Can you work these out from the model? Positions are in its coordinate system, mm. A direction names the side the tool comes from. Give positions to 0.01 mm unless a question says otherwise; leave off trailing zeros. Order: outer loops, then holes, each group sorted by start corner. A loop starts at its lowest first (then second) coordinate and runs counter-clockwise, first axis right, second up. Notation, with made-up numbers: M -6.5,13.5 L 50.5,13.5 A30 cw 50.5,35.5 Z; hole C 0,-32.75 d5. An arc over 180 degrees is marked long. Answer as a JSON object with one key per item and string values.
Autodesk Inventor part; units mm, degrees
ref_plane "Work Plane1" through (-19.6075, -25, -15) normal (0, 0, 1) x (1, 0, 0)
ref_plane "Work Plane2" through (-137.3725, -100, -40) normal (0, 0, -1) x (0, 1, 0)
ref_plane "Work Plane3" through (-19.6075, -25, -15) normal (0, 0, 1) x (1, 0, 0)
sketch "Sketch1" plane through (0, 0, 0) normal (0, 0, 1) x (1, 0, 0)
  circle A0 centre (0, 0) radius 19.4
  circle A1 centre (0, 0) radius 14
  dimension "d0" = 38.8
  dimension "d1" = 28
extrude "Extrusion1" add sketch "Sketch1" against normal blind 2
ref_plane "Work Plane1" through (-19.6075, -25, -15) normal (0, 0, 1) x (1, 0, 0)
ref_plane "Work Plane2" through (-137.3725, -100, -40) normal (0, 0, -1) x (0, 1, 0)
sketch "Sketch5" plane through (0, 0, -2) normal (0, 0, -1) x (-1, 0, 0)
  circle A0 centre (0, 0) radius 19.4
  line L0 (-5.1962, -3) -> (-5.1962, 3)
  line L1 (-5.1962, 3) -> (0, 6)
  line L2 (0, 6) -> (5.1962, 3)
  line L3 (5.1962, 3) -> (5.1962, -3)
  line L4 (5.1962, -3) -> (0, -6)
  line L5 (0, -6) -> (-5.1962, -3)
  dimension "d14" = 6
extrude "Extrusion5" add sketch "Sketch5" along normal blind 3
sketch "Sketch6" plane through (0, 0, -5) normal (0, 0, -1) x (-1, 0, 0)
  circle A0 centre (0, 0) radius 19.4
  line L0 (-5.1962, -3) -> (-5.1962, 3)
  line L1 (-5.1962, 3) -> (0, 6)
  line L2 (0, 6) -> (5.1962, 3)
  line L3 (5.1962, 3) -> (5.1962, -3)
  line L4 (5.1962, -3) -> (0, -6)
  line L5 (0, -6) -> (-5.1962, -3)
  line L6 (-6.1962, 3.5774) -> (-6.1962, -3.5774)
  line L7 (-6.1962, -3.5774) -> (0, -7.1547)
  line L8 (0, -7.1547) -> (6.1962, -3.5774)
  line L9 (6.1962, -3.5774) -> (6.1962, 3.5774)
  line L10 (6.1962, 3.5774) -> (0, 7.1547)
  line L11 (0, 7.1547) -> (-6.1962, 3.5774)
  dimension "d17" = 1
ref_plane "Work Plane3" through (-19.6075, -25, -15) normal (0, 0, 1) x (1, 0, 0)
extrude "Extrusion6" add sketch "Sketch6" along normal up to surface (10 mm away) contours L0 L1 L2 L3 L4 L5 | L11 L10 L9 L8 L7 L6
sketch "Sketch7" plane through (6.1962, -3.5774, -15) normal (0, 0, -1) x (-1, 0, 0)
  circle A0 centre (6.1962, 3.5774) radius 3.75
  dimension "d20" = 7.5
ref_plane "Work Plane4" through (-137.3725, -100, -40) normal (0, 0, -1) x (0, 1, 0)
extrude "Extrusion7" add sketch "Sketch7" along normal up to surface (25 mm away)
properties part number "Reverser"
1) For faces 4 (the face through (3, -3, -15)), 5 (the face through (-3.14, 5.34, -9.93)), 6 (the face through (-6.196, 0, -10)), which set-ups out of +Z, -Z, +X, -X, +Y, -Y let a thin tool reach every point of the face, with its end or its side?
Results found:
{"face 4": "-Z", "face 5": "-Z, -X, +Y", "face 6": "-Z, -X, +Y, -Y"}
2) I want a section at B-B on z = -13.5. Write out the boundary of the cut face in (x, y), and give its area (3 significant figures).
Results found:
{"outline": "M -6.2,-3.58 L 0,-7.15 L 6.2,-3.58 L 6.2,3.58 L 0,7.15 L -6.2,3.58 Z", "area": "133 mm²"}
3) I need wall thicknesses on L1, parallel to Z at x = 5, y = 12.5; L2, parallel to Y at x = 0, z = -1; L3, parallel to Z at x = -13.5, y = 7.5. Which ranges of each line are inside material? Lowest first, please.
Results found:
{"L1": "z = -5 to -2", "L2": "y = -19.4 to -14, 14 to 19.4", "L3": "z = -5 to 0"}
4) I'm going to push flat-ended pins straight in: pin 1 Ø12 at (y, z) = (6, -35) entering from +X; pin 2 Ø2 at (y, z) = (-0.5, -10) entering from -X; pin 3 Ø12 at (x, y) = (10.5, 11) entering from -Z. Where does each tip first touch, or does it pass through?
Results found:
{"pin 1": "stops at x = 3.75", "pin 2": "stops at x = -6.2", "pin 3": "stops at z = -5"}
5) I want a section at A-A on y = 0. Write out the boundary of the cut face in (x, z), and give its area (3 significant figures).
Results found:
{"outline": "M -19.4,-5 L -6.2,-5 L -6.2,-15 L -3.75,-15 L -3.75,-40 L 3.75,-40 L 3.75,-15 L 6.2,-15 L 6.2,-5 L 19.4,-5 L 19.4,0 L 14,0 L 14,-2 L 5.2,-2 L 5.2,-5 L -5.2,-5 L -5.2,-2 L -14,-2 L -14,0 L -19.4,0 Z", "area": "418 mm²"}
6) I want a section at D-D on y = 9. Write out the boundary of the cut face in (x, z).
Results found:
{"outline": "M -17.19,-5 L 17.19,-5 L 17.19,0 L 10.72,0 L 10.72,-2 L -10.72,-2 L -10.72,0 L -17.19,0 Z"}
7) Thinking about a two-plate mould opening in Y: for faces 1 (the face through (-6, 0, -2)), 2 (the face through (3.14, -5.34, -9.93)), 3 (the face through (3.055, 5.391, -9.93)), which applies, pulls with the +Y half, pulls with the -Y half, needs draft (parallel to the pull), parting line crosses it, or undercut?
Results found:
{"face 1": "undercut", "face 2": "pulls with the -Y half", "face 3": "pulls with the +Y half"}
8) I want a section at C-C on x = -2. Write out the boundary of the cut face in (y, z).
Results found:
{"outline": "M -19.3,-5 L -6,-5 L -6,-15 L -3.17,-15 L -3.17,-40 L 3.17,-40 L 3.17,-15 L 6,-15 L 6,-5 L 19.3,-5 L 19.3,0 L 13.86,0 L 13.86,-2 L 4.85,-2 L 4.85,-5 L -4.85,-5 L -4.85,-2 L -13.86,-2 L -13.86,0 L -19.3,0 Z"}
